Design review of the part built by this model. Coordinates are the model's own, in mm. Coordinates: 2 decimals unless noted, no trailing zeros. Loops run counter-clockwise (first coordinate to the right, second up) from the corner with the lowest first, then second, coordinate; pieces in that order, holes last. Notation, with made-up numbers: (55.5, 28.25) -> (81.5, 28.25) arc R16 ccw to (81.5, 42.25) -> close; hole circle Ø6 at (39.25, 87.5). An arc over 180 degrees is marked (long way). Answer in a Markdown table with one row per item.
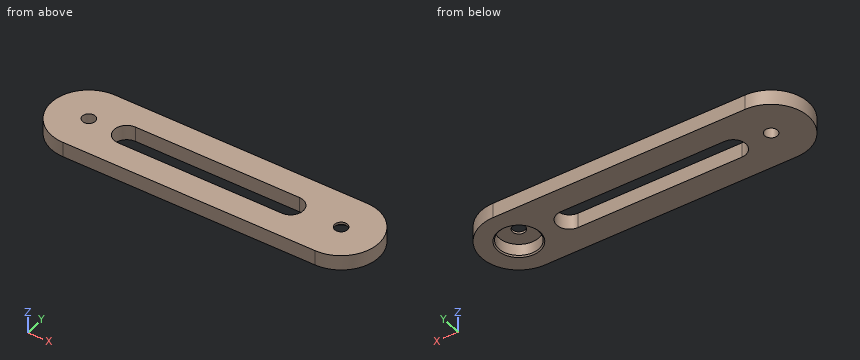
```python
from build123d import *

# Parameters (mm, degrees)
BOSS_EXTRUDE1_DEPTH = 6
SKETCH9_R           = 7.975
CUT_EXTRUDE5_DEPTH  = 5.1
SKETCH10_R          = 2.55
CUT_EXTRUDE6_DEPTH  = 1.9
SKETCH11_R          = 2.55
CUT_EXTRUDE7_DEPTH  = 7
CHAMFER1_SIZE       = 0.5
CUT_EXTRUDE8_DEPTH  = 7


with BuildPart() as part:
    # Sketch4 → Boss-Extrude1 (new body)
    with BuildSketch(Plane.XY):
        with BuildLine():
            Line((-50, 15), (50, 15))
            ThreePointArc((50, 15), (65, 0), (50, -15))
            Line((50, -15), (-50, -15))
            ThreePointArc((-50, -15), (-65, 0), (-50, 15))
        make_face()
    extrude(amount=BOSS_EXTRUDE1_DEPTH)

    # Sketch9 → Cut-Extrude5 (cut)
    with BuildSketch(Plane(origin=(0, 0, 0), x_dir=(-1, 0, 0), z_dir=(0, 0, -1))):
        with Locations((-50, 0)):
            Circle(SKETCH9_R)
    extrude(amount=-CUT_EXTRUDE5_DEPTH, mode=Mode.SUBTRACT)

    # Sketch10 → Cut-Extrude6 (cut, through all)
    with BuildSketch(Plane(origin=(0, 0, 5.1), x_dir=(-1, 0, 0), z_dir=(0, 0, -1))):
        with Locations((-50, 0)):
            Circle(SKETCH10_R)
    extrude(amount=-CUT_EXTRUDE6_DEPTH, mode=Mode.SUBTRACT)

    # Sketch11 → Cut-Extrude7 (cut, through all)
    with BuildSketch(Plane(origin=(0, 0, 0), x_dir=(-1, 0, 0), z_dir=(0, 0, -1))):
        with Locations((50, 0)):
            Circle(SKETCH11_R)
    extrude(amount=-CUT_EXTRUDE7_DEPTH, mode=Mode.SUBTRACT)

    # Chamfer1
    chamfer1_edges = [part.edges().sort_by_distance(p)[0] for p in [
        (57.975, 0, 0),
    ]]
    chamfer(chamfer1_edges, length=CHAMFER1_SIZE)

    # Sketch12 → Cut-Extrude8 (cut, through all)
    with BuildSketch(Plane(origin=(0, 0, 0), x_dir=(-1, 0, 0), z_dir=(0, 0, -1))):
        with BuildLine():
            Line((-30, 5), (35, 5))
            ThreePointArc((35, 5), (40, 0), (35, -5))
            Line((35, -5), (-30, -5))
            ThreePointArc((-30, -5), (-35, 0), (-30, 5))
        make_face()
    extrude(amount=-CUT_EXTRUDE8_DEPTH, mode=Mode.SUBTRACT)


solid = part.part
```
(1) To check wall thickness, follow probe 1 along Y at (x, z) = (50, 3.15) (3 decimals); probe 2 along Y at (x, z) = (50, 5.35); probe 3 along X at (y, z) = (-0.5, 3.3). State the ranges of each line that lie inside material, in increasing order.
Evaluation:
| item | result |
|---|---|
| probe 1 | y = -15 to -7.975, 7.975 to 15 |
| probe 2 | y = -15 to -2.55, 2.55 to 15 |
| probe 3 | x = -64.99 to -52.5, -47.5 to -39.97, 34.97 to 42.04, 57.96 to 64.99 |
(2) Take a section at A-A on x = 7.5. Give the boundary of the cut face in (y, z).
Evaluation:
| item | result |
|---|---|
| outline | (-15, 0) -> (-5, 0) -> (-5, 6) -> (-15, 6) -> close; (5, 0) -> (15, 0) -> (15, 6) -> (5, 6) -> close |
(3) Take a section at D-D on y = -12. Give the boundary of the cut face in (x, z), and give its area (3 significant figures).
Evaluation:
| item | result |
|---|---|
| outline | (-59, 0) -> (59, 0) -> (59, 6) -> (-59, 6) -> close |
| area | 708 mm² |
(4) Take a section at B-B on z = 2.05. Give the boundary of the cut face in (x, y) (3 decimals).
Evaluation:
| item | result |
|---|---|
| outline | (-50, -15) -> (50, -15) arc R15 ccw to (50, 15) -> (-50, 15) arc R15 ccw to start; hole circle Ø5.1 at (-50, 0); hole (-35, -5) -> (30, -5) arc R5 ccw to (30, 5) -> (-35, 5) arc R5 ccw to start; hole circle Ø15.95 at (50, 0) |
(5) Take a section at C-C on y = 0. Give the boundary of the cut face in (x, z) (3 decimals).
Evaluation:
| item | result |
|---|---|
| outline | (-65, 0) -> (-52.55, 0) -> (-52.55, 6) -> (-65, 6) -> close; (-47.45, 0) -> (-40, 0) -> (-40, 6) -> (-47.45, 6) -> close; (35, 0) -> (41.525, 0) -> (42.025, 0.5) -> (42.025, 5.1) -> (47.45, 5.1) -> (47.45, 6) -> (35, 6) -> close; (52.55, 5.1) -> (57.975, 5.1) -> (57.975, 0.5) -> (58.475, 0) -> (65, 0) -> (65, 6) -> (52.55, 6) -> close |
(6) For pin 1 (1.5 mm diameter, centred on y = -9.5, z = 4, fed in from -X); pin 2 (1 mm diameter, centred on y = -10.5, z = 1, fed in from +X); pin 3 (5 mm diameter, centred on x = 49, y = -2.5, fed in from -Z); pin 4 (3 mm diameter, centred on x = 50, y = 0, fed in from -Z), all flat-tipped, find the tip position at first contact; note any pin that passes through.
Evaluation:
| item | result |
|---|---|
| pin 1 | stops at x = -62.18 |
| pin 2 | stops at x = 61.18 |
| pin 3 | stops at z = 5.1 |
| pin 4 | passes through |
